The listing builds one solid part. Answer for the finished solid, in the listing's coordinates (mm). Coordinates: 2 decimals unless noted, no trailing zeros. Write each loop counter-clockwise with the first axis right and the second up, starting at its lowest first coordinate (ties: lowest second). Pieces come first, ordered by that corner, then holes.
(1) The part is cut by section B-B on x = -49.5. Determine the outline of the cut face in (y, z) (3 decimals), plus the area to 3 significant figures.
(2) The part is cut by section C-C on z = -32.5. Determine the outline of the cut face in (x, y) (3 decimals), plus the area to 3 significant figures.
(3) The part is cut by section A-A on y = 2.3. Determine the outline of the cut face in (x, z) (3 decimals).
(4) Given P1, Ø1.5, axis at x = -130.5, y = 1.5, coming from the -Z side; P2, Ø0.5, axis at x = -229.5, y = 2, coming from the -Z side; P3, Ø1, axis at y = 1.5, z = 160, coming from the -X side; P4, Ø3, axis at x = 13.5, z = -31, coming from the -Y side, each flat-ended and moving along its own axis, determine where each tip first touches the part or whether it passes through.
(5) Straight lines are drawn through the part: line 1 (X direction, y = 2.15, z = 16.5); line 2 (Z direction, x = 78.5, y = 1.65); line 3 (Z direction, x = -46.5, y = 1.7). For each, find the intervals that lie inside material, in ascending order.
from build123d import *

# Parameters (mm, degrees)
BOSS_EXTRUDE1_DEPTH     = 3.175
CUT_EXTRUDE1_DEPTH      = 285.023893051
CUT_EXTRUDE1_DEPTH_BACK = 285.023893051


with BuildPart() as part:
    # Sketch1 → Boss-Extrude1 (new body)
    with BuildSketch(Plane(origin=(0, 0, 0), x_dir=(1, 0, 0), z_dir=(0, 1, 0))):
        with BuildLine():
            Line((197.005348369, -26.67), (197.005348369, -163.83))
            Line((197.005348369, -163.83), (176.367848369, -163.83))
            Line((176.367848369, -163.83), (176.367848369, -167.005))
            Line((176.367848369, -167.005), (116.042848369, -167.005))
            Line((116.042848369, -167.005), (116.042848369, -163.83))
            Line((116.042848369, -163.83), (-116.042848369, -163.83))
            Line((-116.042848369, -163.83), (-148.752151631, -163.83))
            Line((-148.752151631, -163.83), (-148.752151631, -167.005))
            Line((-148.752151631, -167.005), (-209.077151631, -167.005))
            Line((-209.077151631, -167.005), (-209.077151631, -163.83))
            Line((-209.077151631, -163.83), (-226.539651631, -163.83))
            Line((-226.539651631, -163.83), (-226.539651631, -157.48))
            ThreePointArc((-226.539651631, -157.48), (-227.283600406, -155.683948776), (-229.079651631, -154.94))
            Line((-229.079651631, -154.94), (-229.714651631, -154.94))
            Line((-229.714651631, -154.94), (-229.714651631, -26.67))
            Line((-229.714651631, -26.67), (-229.079651631, -26.67))
            ThreePointArc((-229.079651631, -26.67), (-227.283600406, -25.926051224), (-226.539651631, -24.13))
            Line((-226.539651631, -24.13), (-226.539651631, 0))
            Line((-226.539651631, 0), (-6.194651631, 0))
            Line((-6.194651631, 0), (-6.194651631, 64.77))
            Line((-6.194651631, 64.77), (193.830348369, 64.77))
            Line((193.830348369, 64.77), (193.830348369, -24.13))
            ThreePointArc((193.830348369, -24.13), (194.574297145, -25.926051224), (196.370348369, -26.67))
            Line((196.370348369, -26.67), (197.005348369, -26.67))
        make_face()
    extrude(amount=BOSS_EXTRUDE1_DEPTH)

    # Sketch2 → Cut-Extrude1 (cut, two sides: drawn at the far end of the back side and taken through both)
    with BuildSketch(Plane(origin=(0, 3.175, 0), x_dir=(1, 0, 0), z_dir=(0, 1, 0)).offset(-CUT_EXTRUDE1_DEPTH_BACK)):
        with BuildLine():
            Line((197.005348369, -163.83), (193.830348369, -163.83))
            Line((193.830348369, -163.83), (193.830348369, -157.48))
            ThreePointArc((193.830348369, -157.48), (194.574297145, -155.683948776), (196.370348369, -154.94))
            Line((196.370348369, -154.94), (197.005348369, -154.94))
            Line((197.005348369, -154.94), (197.005348369, -163.83))
        make_face()
    extrude(amount=CUT_EXTRUDE1_DEPTH + CUT_EXTRUDE1_DEPTH_BACK, mode=Mode.SUBTRACT)


solid = part.part
Model answer:
1. outline: (0, 0) - (3.175, 0) - (3.175, 163.83) - (0, 163.83) - close
1. area: 520 mm2
2. outline: (-6.195, 0) - (193.83, 0) - (193.83, 3.175) - (-6.195, 3.175) - close
2. area: 635 mm2
3. outline: (-229.715, 26.67) - (-229.08, 26.67) arc R2.54 cw to (-226.54, 24.13) - (-226.54, 0) - (-6.195, 0) - (-6.195, -64.77) - (193.83, -64.77) - (193.83, 24.13) arc R2.54 cw to (196.37, 26.67) - (197.005, 26.67) - (197.005, 154.94) - (196.37, 154.94) arc R2.54 cw to (193.83, 157.48) - (193.83, 163.83) - (176.368, 163.83) - (176.368, 167.005) - (116.043, 167.005) - (116.043, 163.83) - (-148.752, 163.83) - (-148.752, 167.005) - (-209.077, 167.005) - (-209.077, 163.83) - (-226.54, 163.83) - (-226.54, 157.48) arc R2.54 cw to (-229.08, 154.94) - (-229.715, 154.94) - close
4. P1: stops at z = 0
4. P2: stops at z = 26.67
4. P3: stops at x = -226.54
4. P4: stops at y = 0
5. line 1: x = -226.54 to 193.83
5. line 2: z = -64.77 to 163.83
5. line 3: z = 0 to 163.83
